```python
from build123d import *

# Parameters (mm, degrees)
ESBO_O1_W                = 30
ESBO_O1_H                = 10
ESBO_O1_W_2              = 26
ESBO_O1_H_2              = 6
RESSALTO_EXTRUS_O1_DEPTH = 80
ESBO_O2_R                = 4
CORTE_EXTRUS_O1_DEPTH    = 10
ESBO_O3_W                = 26
ESBO_O3_H                = 10
CORTE_EXTRUS_O2_DEPTH    = 2
ESBO_O5_W                = 26
ESBO_O5_H                = 10
CORTE_EXTRUS_O3_DEPTH    = 2
ESBO_O6_R                = 2
CORTE_EXTRUS_O4_DEPTH    = 2
ESBO_O7_R                = 1.25
CORTE_EXTRUS_O5_DEPTH    = 2


with BuildPart() as part:
    # Esboço1 → Ressalto-extrusão1 (new body)
    with BuildSketch(Plane.XY):
        with Locations((15, 5)):
            Rectangle(ESBO_O1_W, ESBO_O1_H)
        with Locations((15, 5)):
            Rectangle(ESBO_O1_W_2, ESBO_O1_H_2, mode=Mode.SUBTRACT)
    extrude(amount=RESSALTO_EXTRUS_O1_DEPTH)

    # Esboço2 → Corte-extrusão1 (cut)
    with BuildSketch(Plane(origin=(0, 10, 0), x_dir=(1, 0, 0), z_dir=(0, 1, 0))):
        with Locations(Location((15, -40, 0), (0, 0, 270))):
            Circle(ESBO_O2_R)
    extrude(amount=-CORTE_EXTRUS_O1_DEPTH, mode=Mode.SUBTRACT)

    # Esboço3 → Corte-extrusão2 (cut)
    with BuildSketch(Plane(origin=(0, 10, 0), x_dir=(1, 0, 0), z_dir=(0, 1, 0))):
        with Locations((15, -40)):
            Rectangle(ESBO_O3_W, ESBO_O3_H)
    extrude(amount=-CORTE_EXTRUS_O2_DEPTH, mode=Mode.SUBTRACT)

    # Esboço5 → Corte-extrusão3 (cut)
    with BuildSketch(Plane(origin=(0, 0, 0), x_dir=(-1, 0, 0), z_dir=(0, -1, 0))):
        with Locations((-15, -58.5)):
            Rectangle(ESBO_O5_W, ESBO_O5_H)
    corte_extrus_o3 = extrude(amount=-CORTE_EXTRUS_O3_DEPTH, mode=Mode.SUBTRACT)

    # Esboço6 → Corte-extrusão4 (cut)
    with BuildSketch(Plane(origin=(0, 8, 0), x_dir=(-1, 0, 0), z_dir=(0, -1, 0))):
        with Locations(Location((-15.391952085, -58.25, 0), (0, 0, 90))):
            Circle(ESBO_O6_R)
    corte_extrus_o4 = extrude(amount=-CORTE_EXTRUS_O4_DEPTH, mode=Mode.SUBTRACT)

    # Espelhar6: Corte-extrusão3, Corte-extrusão4 across plane
    add(corte_extrus_o3.mirror(Plane(origin=(0, 0, 40), x_dir=(1, 0, 0), z_dir=(0, 0, -1))), mode=Mode.SUBTRACT)
    add(corte_extrus_o4.mirror(Plane(origin=(0, 0, 40), x_dir=(1, 0, 0), z_dir=(0, 0, -1))), mode=Mode.SUBTRACT)

    # Esboço7 → Corte-extrusão5 (cut)
    with BuildSketch(Plane(origin=(0, 2, 0), x_dir=(1, 0, 0), z_dir=(0, 1, 0))):
        with Locations(Location((24.53, -40, 0), (0, 0, 270))):
            Circle(ESBO_O7_R)
    corte_extrus_o5 = extrude(amount=-CORTE_EXTRUS_O5_DEPTH, mode=Mode.SUBTRACT)

    # Espelhar7: Corte-extrusão5 across plane
    add(corte_extrus_o5.mirror(Plane.ZY.offset(-15)), mode=Mode.SUBTRACT)


solid = part.part
```
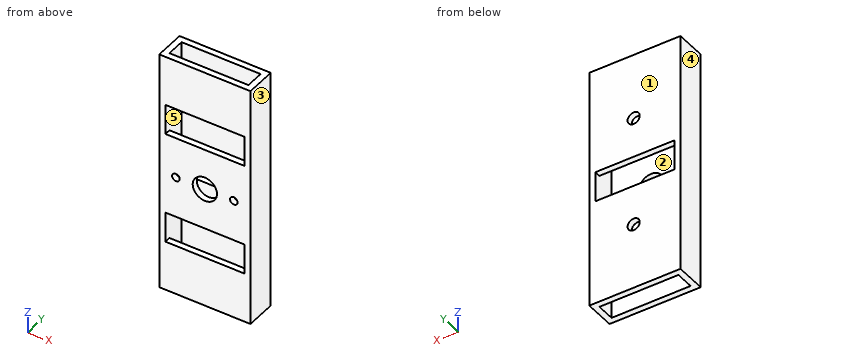
Build history of the part. All positions in model axes, mm. Face numbers are marked on the shaded views. A direction names the side the tool comes from. Give positions to 0.01 mm unless a question says otherwise; leave off trailing zeros. Loops run counter-clockwise (first coordinate to the right, second up) from the corner with the lowest first, then second, coordinate; pieces in that order, holes last.
Item 1: Slice it at D-D, the plane x = 24.53. List the corners of the cut face in (y, z), and give its area (3 significant figures).
Answers follow:
outline: (0, 0) - (2, 0) - (2, 16.5) - (0, 16.5) - close; (0, 26.5) - (2, 26.5) - (2, 38.75) - (0, 38.75) - close; (0, 41.25) - (2, 41.25) - (2, 53.5) - (0, 53.5) - close; (0, 63.5) - (2, 63.5) - (2, 80) - (0, 80) - close; (8, 0) - (10, 0) - (10, 35) - (8, 35) - close; (8, 45) - (10, 45) - (10, 80) - (8, 80) - close
area: 255 mm2
Item 2: Pull direction X, two halves, no side cores. Call the marked faces 3, 4 and 5: released by +X, released by -X, zero draft, split by the parting line, or undercut.
Answers follow:
face 3: released by +X
face 4: released by -X
face 5: undercut
Item 3: Slice it at A-A, the plane z = 40. List the corners of the cut face in (x, y), and give its area (3 significant figures).
Answers follow:
outline: (0, 0) - (4.22, 0) - (4.22, 2) - (2, 2) - (2, 10) - (0, 10) - close; (6.72, 0) - (11, 0) - (11, 2) - (6.72, 2) - close; (19, 0) - (23.28, 0) - (23.28, 2) - (19, 2) - close; (25.78, 0) - (30, 0) - (30, 10) - (28, 10) - (28, 2) - (25.78, 2) - close
area: 66.0 mm2
Item 4: Slice it at C-C, the plane z = 58.25. List the corners of the cut face in (x, y).
Answers follow:
outline: (0, 0) - (2, 0) - (2, 8) - (13.39, 8) - (13.39, 10) - (0, 10) - close; (17.39, 8) - (28, 8) - (28, 0) - (30, 0) - (30, 10) - (17.39, 10) - close
Item 5: Which spindle directions (+Z, -Z, +X, -X, +Y, -Y) get a long thin tool onto all of the face, cutting with end or side? Do the marked faces 1 and 2. Say none if no direction does.
Answers follow:
face 1: +Z, -Z, +X, -X, +Y
face 2: +Z, -Z
Item 6: Drill centre lines: line 1 (Z direction, x = 5.47, y = 1.1); line 2 (X direction, y = 0.8, z = 40); line 3 (X direction, y = 7.5, z = 24). Where is each one in solid material? Low to high.
Answers follow:
line 1: z = 0 to 16.5, 26.5 to 38.75, 41.25 to 53.5, 63.5 to 80
line 2: x = 0 to 4.22, 6.72 to 11, 19 to 23.28, 25.78 to 30
line 3: x = 0 to 2, 28 to 30
Item 7: Slice it at B-B, the plane y = 7.25. List the corners of the cut face in (x, z), and give its area (3 significant figures).
Answers follow:
outline: (0, 0) - (2, 0) - (2, 80) - (0, 80) - close; (28, 0) - (30, 0) - (30, 80) - (28, 80) - close
area: 320 mm2
